from build123d import *

# Parameters (mm, degrees)
CUT_EXTRUDE_1_DEPTH      = 17
CUT_EXTRUDE_1_DEPTH_BACK = 17


with BuildPart() as part:
    # Sketch 1 → Revolve 1 (revolve)
    with BuildSketch(Plane.XY):
        Polygon((0, 0), (0, 10), (60.5, 10), (60.5, 25), (81.5, 25), (81.5, 0), align=None)
    revolve(axis=Axis((81.5, 0, 0), (-1, 0, 0)))

    # Sketch 2 → Revolve 2 (revolve)
    with BuildSketch(Plane.XY):
        Polygon((-33.5, 0), (-33.5, 8.08), (-32.58, 9), (-5, 9), (-4, 10), (0, 10), (0, 0), align=None)
    revolve(axis=Axis((0, 0, 0), (-1, 0, 0)))

    # Sketch 3 → Cut-Extrude 1 (cut, two sides)
    with BuildSketch(Plane(origin=(0, 0, 0), x_dir=(1, 0, 0), z_dir=(0, 1, 0))) as cut_extrude_1_sk:
        Polygon((-43.5, -28.5), (19, -28.5), (-1, -8.5), (-5, -8.5), (-5, -18.5), (-33.5, -18.5), (-33.5, 18.5), (-5, 18.5), (-5, 8.5), (-1, 8.5), (19, 28.5), (-43.5, 28.5), align=None)
    extrude(amount=CUT_EXTRUDE_1_DEPTH, mode=Mode.SUBTRACT)
    extrude(cut_extrude_1_sk.sketch, amount=-CUT_EXTRUDE_1_DEPTH_BACK, mode=Mode.SUBTRACT)


solid = part.part
Design review of the part built by this model. Coordinates are the model's own, in mm. A direction names the side the tool comes from. Round coordinates to 2 decimals unless told otherwise and drop trailing zeros. Write each loop counter-clockwise with the first axis right and the second up, starting at its lowest first coordinate (ties: lowest second). Pieces come first, ordered by that corner, then holes. Notation, with made-up numbers: (-36.5, 12) - (-8.5, 12) arc R21 ccw to (-8.5, 41) - close; hole circle Ø7 at (15, -8.5). An arc over 180 degrees is marked (long way). Return JSON: item names as keys, results as strings. Group by question number.
Item 1: We need section D-D on x = 73. Write out the cut boundary in (y, z), and give its area (3 significant figures).
Item 2: We need section A-A on y = 0. Write out the cut boundary in (x, z), and give its area (3 significant figures).
Item 3: The part is to be moulded in two halves that separate along X. For faces 1 (the face through (-4.8, -9.2, -0.2)), 2 (the face through (81.5, 0, 0)), 3 (the face through (-3, 0, -8.5)), say which applies: pulls with the +X half, pulls with the -X half, needs draft (parallel to the pull), parting line crosses it, or undercut.
Item 4: For probe 1 along X at (y, z) = (7, 20); probe 2 along Y at (x, z) = (33, 0); probe 3 along Z at (x, y) = (38.5, 7), list the stretches that pass through material, from the lowest coordinate up. Write a range as [from, to].
Item 5: Insertion check: P1, Ø4, axis at x = 62, z = 6.5, coming from the +Y side; P2, Ø8, axis at x = 46.5, z = -17.5, coming from the +Y side; P3, Ø1.5, axis at x = 18.5, y = -5.5, coming from the -Z side; P4, Ø5, axis at x = 51.5, y = -1.5, coming from the +Z side. Each pin has a flat end and moves straight along its axis. Give the tip position at first contact, or say it passes through.
Item 6: We need section C-C on x = 22.5. Write out the cut boundary in (y, z).
Item 7: We need section B-B on z = 0. Write out the cut boundary in (x, y).
Item 8: Machinability: for faces 4 (the face through (-4.8, 9.2, 0.2)), 5 (the face through (-3, 0, 8.5)), 6 (the face through (60.5, 0, 11)), which of the approach directions +Z, -Z, +X, -X, +Y, -Y give a long, thin tool a straight path to every point of the face, cutting with its end or side? Answer none if there is none.
Model answer:
{
 "1": {"outline": "circle Ø50 at (0, 0)", "area": "1,960 mm²"},
 "2": {"outline": "(-33.5, -8.08) - (-32.58, -9) - (-5, -9) - (-5, -8.5) - (-1, -8.5) - (0.5, -10) - (60.5, -10) - (60.5, -25) - (81.5, -25) - (81.5, 25) - (60.5, 25) - (60.5, 10) - (0.5, 10) - (-1, 8.5) - (-5, 8.5) - (-5, 9) - (-32.58, 9) - (-33.5, 8.08) - close", "area": "2,860 mm²"},
 "3": {"face 1": "pulls with the -X half", "face 2": "pulls with the +X half", "face 3": "undercut"},
 "4": {"probe 1": "x = [60.5, 81.5]", "probe 2": "y = [-10, 10]", "probe 3": "z = [-7.14, 7.14]"},
 "5": {"P1": "stops at y = 24.59", "P2": "passes through", "P3": "stops at z = -8.8", "P4": "stops at z = 10"},
 "6": {"outline": "circle Ø20 at (0, 0)"},
 "7": {"outline": "(-33.5, -8.08) - (-32.58, -9) - (-5, -9) - (-4, -10) - (60.5, -10) - (60.5, -25) - (81.5, -25) - (81.5, 25) - (60.5, 25) - (60.5, 10) - (-4, 10) - (-5, 9) - (-32.58, 9) - (-33.5, 8.08) - close"},
 "8": {"face 4": "-X, +Y", "face 5": "+Z, +Y, -Y", "face 6": "-X"}
}
